```python
from build123d import *

# Parameters (mm, degrees)
F0_R     = 57.932951026
F0_W     = 2.9168109343
F0_H     = 13.753260226
F1_DEPTH = 12.7


with BuildPart() as f1:
    # F0 (on Front) → F1 (new body)
    with BuildSketch(Plane.XZ):
        Circle(F0_R)
        with BuildLine():
            add(Edge.make_bspline(
                [(-19.6506091277, -8.0144570558), (-20.4302314517, -7.7420407611), (-21.1827626525, -7.7420407611)],
                knots=[0, 0, 0, 1, 1, 1], degree=2))
            add(Edge.make_bspline(
                [(-21.1827626525, -7.7420407611), (-22.8293009199, -7.7420407611), (-23.7323383609, -8.9792020552)],
                knots=[0, 0, 0, 1, 1, 1], degree=2))
            add(Edge.make_bspline(
                [(-23.7323383609, -8.9792020552), (-24.6353758019, -10.2163633494), (-24.6353758019, -12.425794955)],
                knots=[0, 0, 0, 1, 1, 1], degree=2))
            add(Edge.make_bspline(
                [(-24.6353758019, -12.425794955), (-24.6353758019, -17.0252656543), (-21.1827626525, -17.0252656543)],
                knots=[0, 0, 0, 1, 1, 1], degree=2))
            add(Edge.make_bspline(
                [(-21.1827626525, -17.0252656543), (-19.7348926222, -17.0252656543), (-17.6759672568, -16.3028357015)],
                knots=[0, 0, 0, 1, 1, 1], degree=2))
            Line((-17.6759672568, -16.3028357015), (-17.6759672568, -18.7470570418))
            add(Edge.make_bspline(
                [(-17.6759672568, -18.7470570418), (-19.3676573962, -19.4544363705), (-21.4566840096, -19.4544363705)],
                knots=[0, 0, 0, 1, 1, 1], degree=2))
            add(Edge.make_bspline(
                [(-21.4566840096, -19.4544363705), (-24.4577784385, -19.4544363705), (-26.0471243346, -17.6333108646)],
                knots=[0, 0, 0, 1, 1, 1], degree=2))
            add(Edge.make_bspline(
                [(-26.0471243346, -17.6333108646), (-27.6364702307, -15.8121853586), (-27.6364702307, -12.4077342061)],
                knots=[0, 0, 0, 1, 1, 1], degree=2))
            add(Edge.make_bspline(
                [(-27.6364702307, -12.4077342061), (-27.6364702307, -10.2615152214), (-26.8553428443, -8.6480883269)],
                knots=[0, 0, 0, 1, 1, 1], degree=2))
            add(Edge.make_bspline(
                [(-26.8553428443, -8.6480883269), (-26.0742154578, -7.0346614323), (-24.6112948034, -6.175270801)],
                knots=[0, 0, 0, 1, 1, 1], degree=2))
            add(Edge.make_bspline(
                [(-24.6112948034, -6.175270801), (-23.1483741491, -5.3158801697), (-21.1827626525, -5.3158801697)],
                knots=[0, 0, 0, 1, 1, 1], degree=2))
            add(Edge.make_bspline(
                [(-21.1827626525, -5.3158801697), (-19.1810296584, -5.3158801697), (-17.1582257906, -6.2821302315)],
                knots=[0, 0, 0, 1, 1, 1], degree=2))
            Line((-17.1582257906, -6.2821302315), (-18.0973847292, -8.6541085765))
            add(Edge.make_bspline(
                [(-18.0973847292, -8.6541085765), (-18.8709868037, -8.2868733505), (-19.6506091277, -8.0144570558)],
                knots=[0, 0, 0, 1, 1, 1], degree=2))
        make_face(mode=Mode.SUBTRACT)
        with BuildLine():
            add(Edge.make_bspline(
                [(-3.9467880292, -7.1204499892), (-2.267138389, -8.9460906824), (-2.267138389, -12.3686025837)],
                knots=[0, 0, 0, 1, 1, 1], degree=2))
            add(Edge.make_bspline(
                [(-2.267138389, -12.3686025837), (-2.267138389, -15.7850942354), (-3.9603335908, -17.619765303)],
                knots=[0, 0, 0, 1, 1, 1], degree=2))
            add(Edge.make_bspline(
                [(-3.9603335908, -17.619765303), (-5.6535287926, -19.4544363705), (-8.814159836, -19.4544363705)],
                knots=[0, 0, 0, 1, 1, 1], degree=2))
            add(Edge.make_bspline(
                [(-8.814159836, -19.4544363705), (-11.9747908794, -19.4544363705), (-13.6679860812, -17.619765303)],
                knots=[0, 0, 0, 1, 1, 1], degree=2))
            add(Edge.make_bspline(
                [(-13.6679860812, -17.619765303), (-15.3611812831, -15.7850942354), (-15.3611812831, -12.3505418349)],
                knots=[0, 0, 0, 1, 1, 1], degree=2))
            add(Edge.make_bspline(
                [(-15.3611812831, -12.3505418349), (-15.3611812831, -8.9159894344), (-13.663470894, -7.1053993652)],
                knots=[0, 0, 0, 1, 1, 1], degree=2))
            add(Edge.make_bspline(
                [(-13.663470894, -7.1053993652), (-11.965760505, -5.2948092961), (-8.7960990872, -5.2948092961)],
                knots=[0, 0, 0, 1, 1, 1], degree=2))
            add(Edge.make_bspline(
                [(-8.7960990872, -5.2948092961), (-5.6264376694, -5.2948092961), (-3.9467880292, -7.1204499892)],
                knots=[0, 0, 0, 1, 1, 1], degree=2))
        make_face(mode=Mode.SUBTRACT)
        with Locations((2.0418552669, -12.3881683949)):
            Rectangle(F0_W, F0_H, mode=Mode.SUBTRACT)
        with BuildLine():
            Line((19.1619400853, -5.5115382819), (19.1619400853, -19.2647985079))
            Line((19.1619400853, -19.2647985079), (15.4564764525, -19.2647985079))
            Line((15.4564764525, -19.2647985079), (9.4723483437, -8.8618071879))
            Line((9.4723483437, -8.8618071879), (9.3880648492, -8.8618071879))
            add(Edge.make_bspline(
                [(9.3880648492, -8.8618071879), (9.5686723374, -11.6160713829), (9.5686723374, -12.793030181)],
                knots=[0, 0, 0, 1, 1, 1], degree=2))
            Line((9.5686723374, -12.793030181), (9.5686723374, -19.2647985079))
            Line((9.5686723374, -19.2647985079), (6.9619042578, -19.2647985079))
            Line((6.9619042578, -19.2647985079), (6.9619042578, -5.5115382819))
            Line((6.9619042578, -5.5115382819), (10.6402767673, -5.5115382819))
            Line((10.6402767673, -5.5115382819), (16.612364377, -15.8121853586))
            Line((16.612364377, -15.8121853586), (16.6785871226, -15.8121853586))
            add(Edge.make_bspline(
                [(16.6785871226, -15.8121853586), (16.5371112569, -13.1301641589), (16.5371112569, -12.0224382313)],
                knots=[0, 0, 0, 1, 1, 1], degree=2))
            Line((16.5371112569, -12.0224382313), (16.5371112569, -5.5115382819))
            Line((16.5371112569, -5.5115382819), (19.1619400853, -5.5115382819))
        make_face(mode=Mode.SUBTRACT)
        Polygon((-18.5308427009, 6.9353277795), (-27.0254148956, 6.9353277795), (-27.0254148956, 20.6885880055), (-24.1086039613, 20.6885880055), (-24.1086039613, 9.3434276221), (-18.5308427009, 9.3434276221), align=None, mode=Mode.SUBTRACT)
        with BuildLine():
            Line((-7.8539300238, 20.6885880055), (-4.9461494639, 20.6885880055))
            Line((-4.9461494639, 20.6885880055), (-4.9461494639, 11.7906590871))
            add(Edge.make_bspline(
                [(-4.9461494639, 11.7906590871), (-4.9461494639, 10.2645258119), (-5.6279427318, 9.1176682619)],
                knots=[0, 0, 0, 1, 1, 1], degree=2))
            add(Edge.make_bspline(
                [(-5.6279427318, 9.1176682619), (-6.3097359997, 7.9708107118), (-7.5995744779, 7.3582503144)],
                knots=[0, 0, 0, 1, 1, 1], degree=2))
            add(Edge.make_bspline(
                [(-7.5995744779, 7.3582503144), (-8.8894129561, 6.7456899169), (-10.6473258412, 6.7456899169)],
                knots=[0, 0, 0, 1, 1, 1], degree=2))
            add(Edge.make_bspline(
                [(-10.6473258412, 6.7456899169), (-13.2992457928, 6.7456899169), (-14.7666816344, 8.106266328)],
                knots=[0, 0, 0, 1, 1, 1], degree=2))
            add(Edge.make_bspline(
                [(-14.7666816344, 8.106266328), (-16.234117476, 9.466842739), (-16.234117476, 11.8267805848)],
                knots=[0, 0, 0, 1, 1, 1], degree=2))
            Line((-16.234117476, 11.8267805848), (-16.234117476, 20.6885880055))
            Line((-16.234117476, 20.6885880055), (-13.3293470409, 20.6885880055))
            Line((-13.3293470409, 20.6885880055), (-13.3293470409, 12.2692689308))
            add(Edge.make_bspline(
                [(-13.3293470409, 12.2692689308), (-13.3293470409, 10.6799230347), (-12.6896955202, 9.9364222083)],
                knots=[0, 0, 0, 1, 1, 1], degree=2))
            add(Edge.make_bspline(
                [(-12.6896955202, 9.9364222083), (-12.0500439995, 9.1929213819), (-10.5720727211, 9.1929213819)],
                knots=[0, 0, 0, 1, 1, 1], degree=2))
            add(Edge.make_bspline(
                [(-10.5720727211, 9.1929213819), (-9.1422634396, 9.1929213819), (-8.4980967317, 9.9409373955)],
                knots=[0, 0, 0, 1, 1, 1], degree=2))
            add(Edge.make_bspline(
                [(-8.4980967317, 9.9409373955), (-7.8539300238, 10.6889534091), (-7.8539300238, 12.2873296797)],
                knots=[0, 0, 0, 1, 1, 1], degree=2))
            Line((-7.8539300238, 12.2873296797), (-7.8539300238, 20.6885880055))
        make_face(mode=Mode.SUBTRACT)
        with BuildLine():
            add(Edge.make_bspline(
                [(5.7969859589, 18.1856692316), (5.0173636349, 18.4580855263), (4.2648324341, 18.4580855263)],
                knots=[0, 0, 0, 1, 1, 1], degree=2))
            add(Edge.make_bspline(
                [(4.2648324341, 18.4580855263), (2.6182941667, 18.4580855263), (1.7152567257, 17.2209242322)],
                knots=[0, 0, 0, 1, 1, 1], degree=2))
            add(Edge.make_bspline(
                [(1.7152567257, 17.2209242322), (0.8122192848, 15.983762938), (0.8122192848, 13.7743313325)],
                knots=[0, 0, 0, 1, 1, 1], degree=2))
            add(Edge.make_bspline(
                [(0.8122192848, 13.7743313325), (0.8122192848, 9.1748606331), (4.2648324341, 9.1748606331)],
                knots=[0, 0, 0, 1, 1, 1], degree=2))
            add(Edge.make_bspline(
                [(4.2648324341, 9.1748606331), (5.7127024644, 9.1748606331), (7.7716278298, 9.8972905859)],
                knots=[0, 0, 0, 1, 1, 1], degree=2))
            Line((7.7716278298, 9.8972905859), (7.7716278298, 7.4530692457))
            add(Edge.make_bspline(
                [(7.7716278298, 7.4530692457), (6.0799376904, 6.7456899169), (3.990911077, 6.7456899169)],
                knots=[0, 0, 0, 1, 1, 1], degree=2))
            add(Edge.make_bspline(
                [(3.990911077, 6.7456899169), (0.9898166481, 6.7456899169), (-0.599529248, 8.5668154229)],
                knots=[0, 0, 0, 1, 1, 1], degree=2))
            add(Edge.make_bspline(
                [(-0.599529248, 8.5668154229), (-2.1888751441, 10.3879409288), (-2.1888751441, 13.7923920813)],
                knots=[0, 0, 0, 1, 1, 1], degree=2))
            add(Edge.make_bspline(
                [(-2.1888751441, 13.7923920813), (-2.1888751441, 15.938611066), (-1.4077477576, 17.5520379605)],
                knots=[0, 0, 0, 1, 1, 1], degree=2))
            add(Edge.make_bspline(
                [(-1.4077477576, 17.5520379605), (-0.6266203712, 19.1654648551), (0.8363002832, 20.0248554864)],
                knots=[0, 0, 0, 1, 1, 1], degree=2))
            add(Edge.make_bspline(
                [(0.8363002832, 20.0248554864), (2.2992209376, 20.8842461177), (4.2648324341, 20.8842461177)],
                knots=[0, 0, 0, 1, 1, 1], degree=2))
            add(Edge.make_bspline(
                [(4.2648324341, 20.8842461177), (6.2665654282, 20.8842461177), (8.289369296, 19.9179960559)],
                knots=[0, 0, 0, 1, 1, 1], degree=2))
            Line((8.289369296, 19.9179960559), (7.3502103574, 17.5460177109))
            add(Edge.make_bspline(
                [(7.3502103574, 17.5460177109), (6.576608283, 17.9132529369), (5.7969859589, 18.1856692316)],
                knots=[0, 0, 0, 1, 1, 1], degree=2))
        make_face(mode=Mode.SUBTRACT)
        Polygon((16.9254173565, 14.6021156534), (21.7596777905, 6.9353277795), (18.448540507, 6.9353277795), (14.8454211175, 12.7298180257), (13.6142800729, 11.8448413336), (13.6142800729, 6.9353277795), (10.6974691386, 6.9353277795), (10.6974691386, 20.6885880055), (13.6142800729, 20.6885880055), (13.6142800729, 14.3944170419), (14.761137623, 16.0138641861), (18.4876721294, 20.6885880055), (21.7235562929, 20.6885880055), align=None, mode=Mode.SUBTRACT)
        Polygon((24.9203088339, 20.6885880055), (27.7708970226, 15.0265432506), (30.6395459601, 20.6885880055), (33.7821162547, 20.6885880055), (29.218767053, 12.2873296797), (29.218767053, 6.9353277795), (26.3230269922, 6.9353277795), (26.3230269922, 12.1940158108), (21.7596777905, 20.6885880055), align=None, mode=Mode.SUBTRACT)
    extrude(amount=F1_DEPTH)


solid = f1.part
```
Geometry: final body of the model. Coordinates: model frame, mm. A direction names the side the tool comes from. Give positions to 0.01 mm unless a question says otherwise; leave off trailing zeros. Write each loop counter-clockwise with the first axis right and the second up, starting at its lowest first coordinate (ties: lowest second). Pieces come first, ordered by that corner, then holes.
1. Reachability of faces 3 (the flat face through (-1, -12.7, 1)), 4 (the flat face through (2, -6, -5.512)) from +Z, -Z, +X, -X, +Y, -Y: full face, straight path, thin tool, end or side. Return the list, or none.
2. Line query: probe 1 along Z at (x, y) = (13, -8.5); probe 2 along Z at (x, y) = (2, -8); probe 3 along Z at (x, y) = (-11.5, -9.5). Output: solid intervals per line, ascending.
3. Section query A-A, the plane x = -12. Count the separate pieces of the cut face and the enclosed holes in it, then the cut area to 3 significant figures.
4. Section query D-D, the plane x = -30. Return loops of the section in (y, z).
5. Section query C-C, the plane z = -42. Return loops of the section in (x, y).
6. Pin query (flat end, axial travel): P1, Ø1, axis at y = -5, z = -4, coming from the -X side; P2, Ø1.6, axis at x = 23.5, y = -8.5, coming from the -Z side; P3, Ø1.5, axis at x = 2.5, y = -3.5, coming from the +Z side; P4, Ø1, axis at x = -37.5, z = -20.5, coming from the +Y side. Return the tip coordinate at first contact, or that it passes through.
7. Draft query along X for faces 1 (the flat face through (-1, 0, 1)), 2 (the flat face through (-27.025, -6, 14)). Return one class per face: released by +X, released by -X, zero draft, split by the parting line, or undercut.
Computed:
1. face 3: +Z, -Z, +X, -X, -Y
1. face 4: +Y, -Y
2. probe 1: z = -56.46 to -14.99, -9.58 to 6.94, 20.69 to 56.46
2. probe 2: z = -57.9 to -19.26, -5.51 to 6.99, 9.96 to 17.56, 20.55 to 57.9
2. probe 3: z = -56.78 to -19.04, -5.71 to 6.78, 9.28 to 56.78
3. separate pieces: 3
3. enclosed holes: 0
3. area: 1,240 mm2
4. outline: (-12.7, -49.56) - (0, -49.56) - (0, 49.56) - (-12.7, 49.56) - close
5. outline: (-39.9, -12.7) - (39.9, -12.7) - (39.9, 0) - (-39.9, 0) - close
6. P1: stops at x = -57.83
6. P2: stops at z = -53.3
6. P3: stops at z = 57.91
6. P4: stops at y = 0
7. face 1: zero draft
7. face 2: undercut
